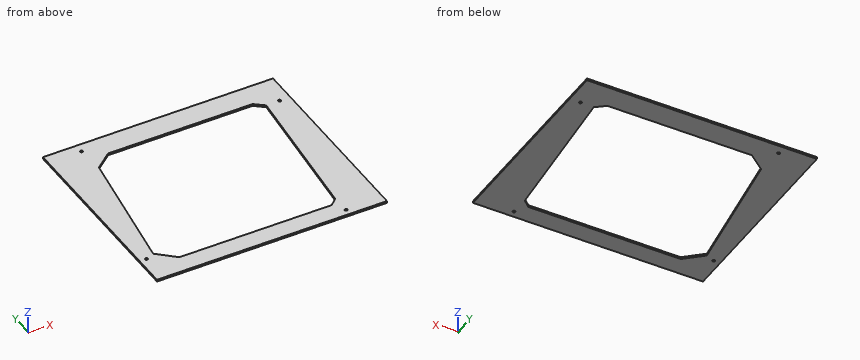
```python
from build123d import *

# Parameters (mm, degrees)
SKETCH1_W           = 346
SKETCH1_H           = 304
SKETCH1_R           = 2
BOSS_EXTRUDE1_DEPTH = 3


with BuildPart() as part:
    # Sketch1 → Boss-Extrude1 (new body)
    with BuildSketch(Plane.XY):
        with Locations((3, 0)):
            Rectangle(SKETCH1_W, SKETCH1_H)
        with Locations((-160, -106)):
            Circle(SKETCH1_R, mode=Mode.SUBTRACT)
        Polygon((108.608210557, -124), (-120.566987488, -124), (-146.683245886, -100.495367441), (-117.140423658, 96.746416259), (-91.823443982, 117), (125.439846228, 117), (139.655171099, 105.627740104), (119.302480143, -114.375157373), align=None, mode=Mode.SUBTRACT)
        with Locations((120, -142)):
            Circle(SKETCH1_R, mode=Mode.SUBTRACT)
        with Locations((-120, 138)):
            Circle(SKETCH1_R, mode=Mode.SUBTRACT)
        with Locations((160, 106)):
            Circle(SKETCH1_R, mode=Mode.SUBTRACT)
    extrude(amount=BOSS_EXTRUDE1_DEPTH)


solid = part.part
```
Design review of the part built by this model. Coordinates are the model's own, in mm. Give positions to 0.01 mm unless a question says otherwise; leave off trailing zeros. Order: outer loops, then holes, each group sorted by start corner. A loop starts at its lowest first (then second) coordinate and runs counter-clockwise, first axis right, second up. Notation, with made-up numbers: M 87,-3 L 145,-3 A17 ccw 145,5 Z; hole C 41,36.25 d2. An arc over 180 degrees is marked long. One line per question, with ' | ' between items. Start each with the question number.
Q1. We need section A-A (x = -78.5). Write out the cut boundary in (y, z).
Q2. We need section B-B (z = 0.9). Write out the cut boundary in (x, y), plus the area to 3 significant figures.
Q3. For pin 1 Ø5 at (x, y) = (-160, -106) entering from +Z, flat-tipped, find the tip position at first contact; note if it passes through.
Q4. For L1, parallel to Y at x = -91, z = 0.6; L2, parallel to X at y = 138, z = 2.3; L3, parallel to X at y = -142, z = 1.6, list the stretches that pass through material, from the lowest coordinate up. Write a range as [from, to].
Returned:
1) outline: M -152,0 L -124,0 L -124,3 L -152,3 Z; M 117,0 L 152,0 L 152,3 L 117,3 Z
2) outline: M -170,-152 L 176,-152 L 176,152 L -170,152 Z; hole C -160,-106 d4; hole M -146.68,-100.5 L -120.57,-124 L 108.61,-124 L 119.3,-114.38 L 139.66,105.63 L 125.44,117 L -91.82,117 L -117.14,96.75 Z; hole C -120,138 d4; hole C 120,-142 d4; hole C 160,106 d4 | area: 42,800 mm2
3) pin 1: z = 3
4) L1: [-152, -124], [117, 152] | L2: [-170, -122], [-118, 176] | L3: [-170, 118], [122, 176]
